```python
from build123d import *

# Parameters (mm, degrees)
SKETCH1_W               = 90
SKETCH1_H               = 25
BOSS_EXTRUDE1_DEPTH     = 20
CUT_EXTRUDE1_DEPTH      = 62.491869381
CUT_EXTRUDE1_DEPTH_BACK = 62.491869381
SKETCH2_W               = 10
SKETCH2_H               = 10
CUT_EXTRUDE2_DEPTH      = 5
CUT_EXTRUDE3_DEPTH      = 62.491869381
HOLE1_D                 = 4.5
LPATTERN1_COUNT         = 2
LPATTERN1_PITCH         = 15
LPATTERN1_COL_COUNT     = 2
LPATTERN1_COL_PITCH     = 60
MIRROR2_COPY_1_D        = 4.5
MIRROR2_COPY_2_D        = 4.5
MIRROR2_COPY_3_D        = 4.5
HOLE2_D                 = 4.5


with BuildPart() as part:
    # Sketch1 → Boss-Extrude1 (new, symmetric)
    with BuildSketch(Plane.XY):
        Rectangle(SKETCH1_W, SKETCH1_H)
    extrude(amount=BOSS_EXTRUDE1_DEPTH, both=True)

    # Sketch2 → Cut-Extrude1 (cut, two sides: drawn at the far end of the back side and taken through both)
    with BuildSketch(Plane.XY.offset(20).offset(-CUT_EXTRUDE1_DEPTH_BACK)):
        with Locations((-40, 7.5)):
            Rectangle(SKETCH2_W, SKETCH2_H)
        with Locations((40, 7.5)):
            Rectangle(SKETCH2_W, SKETCH2_H)
    extrude(amount=CUT_EXTRUDE1_DEPTH + CUT_EXTRUDE1_DEPTH_BACK, mode=Mode.SUBTRACT)

    # Sketch3 → Cut-Extrude2 (cut)
    with BuildSketch(Plane.XY.offset(20)):
        with BuildLine():
            Line((45, -12.5), (45, 2.5))
            Line((45, 2.5), (35, 2.5))
            Line((35, 2.5), (35, 12.5))
            Line((35, 12.5), (30, 12.5))
            ThreePointArc((30, 12.5), (26.338834765, 3.661165235), (17.5, 0))
            Line((17.5, 0), (7.5, 0))
            Line((7.5, 0), (7.5, -12.5))
            Line((7.5, -12.5), (45, -12.5))
        make_face()
        with BuildLine():
            Line((-7.5, -12.5), (-45, -12.5))
            Line((-45, -12.5), (-45, 2.5))
            Line((-45, 2.5), (-35, 2.5))
            Line((-35, 2.5), (-35, 12.5))
            Line((-35, 12.5), (-30, 12.5))
            ThreePointArc((-30, 12.5), (-26.338834765, 3.661165235), (-17.5, 0))
            Line((-17.5, 0), (-7.5, 0))
            Line((-7.5, 0), (-7.5, -12.5))
        make_face()
    cut_extrude2 = extrude(amount=-CUT_EXTRUDE2_DEPTH, mode=Mode.SUBTRACT)

    # Mirror1: Cut-Extrude2 across plane
    add(cut_extrude2.mirror(Plane.XY), mode=Mode.SUBTRACT)

    # Sketch4 → Cut-Extrude3 (cut, through all)
    with BuildSketch(Plane.XY.offset(20)):
        with BuildLine():
            Line((25, 12.5), (10, 12.5))
            ThreePointArc((10, 12.5), (17.5, 5), (25, 12.5))
        make_face()
        with BuildLine():
            Line((-10, 12.5), (-25, 12.5))
            ThreePointArc((-25, 12.5), (-17.5, 5), (-10, 12.5))
        make_face()
    extrude(amount=-CUT_EXTRUDE3_DEPTH, mode=Mode.SUBTRACT)

    # Hole1 (through all)
    with Locations(Plane(origin=(0, 12.5, 0), x_dir=(1, 0, 0), z_dir=(0, 1, 0))):
        with Locations((30, -7.5)):
            hole1 = Hole(HOLE1_D / 2)

    # LPattern1: Hole1 ×2
    with Locations(*[(0, 0, -i * LPATTERN1_PITCH) for i in range(1, LPATTERN1_COUNT)]):
        add(hole1, mode=Mode.SUBTRACT)

    # LPattern1 col: Hole1 ×2
    with Locations(*[(-i * LPATTERN1_COL_PITCH, 0, 0) for i in range(1, LPATTERN1_COL_COUNT)]):
        add(hole1, mode=Mode.SUBTRACT)

    # Mirror2 copy 1 (through all)
    with Locations(Plane(origin=(0, 12.5, -15), x_dir=(-1, 0, 0), z_dir=(0, 1, 0))):
        with Locations((30, 7.5)):
            Hole(MIRROR2_COPY_1_D / 2)

    # Mirror2 copy 2 (through all)
    with Locations(Plane(origin=(60, 12.5, 0), x_dir=(-1, 0, 0), z_dir=(0, 1, 0))):
        with Locations((30, 7.5)):
            Hole(MIRROR2_COPY_2_D / 2)

    # Mirror2 copy 3 (through all)
    with Locations(Plane(origin=(0, 12.5, 0), x_dir=(-1, 0, 0), z_dir=(0, 1, 0))):
        with Locations((30, 7.5)):
            Hole(MIRROR2_COPY_3_D / 2)

    # Hole2 (through all)
    with Locations(Plane(origin=(0, 12.5, 0), x_dir=(1, 0, 0), z_dir=(0, 1, 0))):
        with Locations((0, -15), (0, 15)):
            Hole(HOLE2_D / 2)


solid = part.part
```
The listing builds one solid part. Answer for the finished solid, in the listing's coordinates (mm). A direction names the side the tool comes from. Give positions to 0.01 mm unless a question says otherwise; leave off trailing zeros. Order: outer loops, then holes, each group sorted by start corner. A loop starts at its lowest first (then second) coordinate and runs counter-clockwise, first axis right, second up.
Item 1: The part is cut by section A-A, the plane z = 7.5. Give the vertices of the cut face in (x, y).
From the geometry:
outline: (-45, -12.5) - (-32.25, -12.5) - (-32.25, 12.5) - (-35, 12.5) - (-35, 2.5) - (-45, 2.5) - close; (-27.75, -12.5) - (27.75, -12.5) - (27.75, 12.5) - (25, 12.5) arc R7.5 cw to (10, 12.5) - (-10, 12.5) arc R7.5 cw to (-25, 12.5) - (-27.75, 12.5) - close; (32.25, -12.5) - (45, -12.5) - (45, 2.5) - (35, 2.5) - (35, 12.5) - (32.25, 12.5) - close
Item 2: Find the intervals of material crossed by probe 1 along Z at (x, y) = (30, 1.5); probe 2 along Z at (x, y) = (-0.5, 7.75); probe 3 along X at (y, z) = (-11, -6.5), in increasing order.
From the geometry:
probe 1: z = -15 to -9.75, -5.25 to 5.25, 9.75 to 15
probe 2: z = -20 to -17.19, -12.81 to 12.81, 17.19 to 20
probe 3: x = -45 to -32.02, -27.98 to 27.98, 32.02 to 45
Item 3: For a pull along X with two mould halves and no side action, classify faces 1 (the face through (-7.5, -6, 18)), 2 (the face through (27.854, -0.175, -8.176)), 3 (the face through (-1, -12.5, 0)) as pulls with the +X half, pulls with the -X half, needs draft (parallel to the pull), parting line crosses it, or undercut.
From the geometry:
face 1: pulls with the -X half
face 2: undercut
face 3: needs draft
Item 4: The part is cut by section D-D, the plane x = -16. Give the vertices of the cut face in (y, z), and give its area (3 significant figures).
From the geometry:
outline: (-12.5, -15) - (0, -15) - (0, -20) - (5.15, -20) - (5.15, 20) - (0, 20) - (0, 15) - (-12.5, 15) - close
area: 581 mm2
Item 5: Which of the six approach directions +Z, -Z, +X, -X, +Y, -Y give full straight-line access (tool end or side, diameter ignored) to faces 4 (the face through (-26, -3, -15)), 5 (the face through (-26.435, 3.759, 17.535)), 6 (the face through (-31.21, -0.175, 5.603)), 7 (the face through (26.435, 3.759, 17.535)), 8 (the face through (26.435, 3.759, -17.535))?
From the geometry:
face 4: -Z, -X, -Y
face 5: +Z, -X, -Y
face 6: +Y, -Y
face 7: +Z, +X, -Y
face 8: -Z, +X, -Y
Item 6: The part is cut by section C-C, the plane y = 9.25. Count the separate pieces of the cut face and the enclosed holes in it, and give its area (3 significant figures).
From the geometry:
separate pieces: 3
enclosed holes: 6
area: 1,510 mm2
Item 7: Given pin 1 Ø1 at (y, z) = (5, 3.5) entering from +X; pin 2 Ø6 at (x, y) = (35.5, 5) entering from +Z; pin 3 Ø2 at (x, y) = (-31.5, 6.5) entering from -Z, each flat-ended and moving along its own axis, determine where each tip first touches the part or whether it passes through.
From the geometry:
pin 1: stops at x = 35
pin 2: stops at z = 15
pin 3: stops at z = -15
Item 8: The part is cut by section B-B, the plane y = -9.75. Give the vertices of the cut face in (x, z).
From the geometry:
outline: (-45, -15) - (-7.5, -15) - (-7.5, -20) - (7.5, -20) - (7.5, -15) - (45, -15) - (45, 15) - (7.5, 15) - (7.5, 20) - (-7.5, 20) - (-7.5, 15) - (-45, 15) - close; hole circle Ø4.5 at (-30, -7.5); hole circle Ø4.5 at (-30, 7.5); hole circle Ø4.5 at (0, -15); hole circle Ø4.5 at (0, 15); hole circle Ø4.5 at (30, -7.5); hole circle Ø4.5 at (30, 7.5)
